Read the model definition and answer for the solid it produces. Units are mm, in the model's axes. A direction names the side the tool comes from. Coordinates: 2 decimals unless noted, no trailing zeros. Order: outer loops, then holes, each group sorted by start corner. A loop starts at its lowest first (then second) coordinate and runs counter-clockwise, first axis right, second up. Notation, with made-up numbers: (44, -15) - (99, -15) arc R21 ccw to (99, 1) - close; hole circle Ø5 at (-12, 15.5). An arc over 180 degrees is marked (long way). Use one line per item in the form item = value.
Autodesk Inventor part; units mm, degrees
ref_plane "YZ Plane" through (0, 0, 0) normal (1, 0, 0) x (0, 1, 0)
ref_plane "XZ Plane" through (0, 0, 0) normal (0, 1, 0) x (-1, 0, 0)
ref_plane "XY Plane" through (0, 0, 0) normal (0, 0, 1) x (1, 0, 0)
sketch "Sketch1" plane through (0, 0, 0) normal (0, 1, 0) x (-1, 0, 0)
  line L0 (0, 0) -> (-59, 0)
  line L1 (-59, 0) -> (-59, 5)
  line L2 (-59, 5) -> (0, 5)
  line L3 (0, 5) -> (0, 0)
  line L4 (0, 5) -> (-5, 5)
  line L5 (-5, 5) -> (-5, 47)
  line L6 (-5, 47) -> (0, 47)
  line L7 (0, 47) -> (0, 5)
  line L8 (-59, 5) -> (-54, 5)
  line L9 (-54, 5) -> (-54, 47)
  line L10 (-54, 47) -> (-59, 47)
  line L11 (-59, 47) -> (-59, 5)
  point P0 (-54, 5)
  dimension "d0" = 59
  dimension "d1" = 5
  dimension "d2" = 5
  dimension "d3" = 42
  dimension "d4" = 5
  dimension "d5" = 42
extrude "Extrusion1" add sketch "Sketch1" against normal blind 62
sketch "Sketch7" plane through (0, -62, 0) normal (0, -1, 0) x (1, 0, 0)
  line L0 (0, 47) -> (0, 0)
  line L1 (0, 47) -> (-5, 47)
  line L2 (-5, 47) -> (-5, -5)
  line L3 (-5, -5) -> (0, -5)
  line L4 (0, -5) -> (0, 47)
  line L5 (59, 47) -> (54, 47)
  line L6 (59, 47) -> (64, 47)
  line L7 (64, 47) -> (64, -5)
  line L8 (64, -5) -> (59, -5)
  line L9 (59, -5) -> (59, 47)
  line L10 (0, 0) -> (59, 0)
  line L11 (59, -5) -> (0, -5)
  line L12 (0, -5) -> (0, 0)
  line L13 (0, 0) -> (59, 0)
  line L14 (59, 0) -> (59, -5)
  dimension "d34" = 5
  dimension "d35" = 52
  dimension "d36" = 5
  dimension "d37" = 52
extrude "Extrusion7" add sketch "Sketch7" against normal blind 6
sketch "Sketch8" plane through (0, -62, 0) normal (0, -1, 0) x (1, 0, 0)
  line L0 (0, 0) -> (0, 47)
  line L1 (5, 47) -> (-5, 47)
  circle A0 centre (0, 37) radius 2.5
  line L2 (59, 47) -> (59, 0)
  line L3 (64, 47) -> (54, 47)
  circle A1 centre (59, 37) radius 2.5
  line L4 (59, 0) -> (0, 0)
  line L5 (-5, 47) -> (-5, -5)
  line L6 (64, -5) -> (64, 47)
  circle A2 centre (16.5, 0) radius 2.5
  circle A3 centre (42.5, 0) radius 2.5
  point P0 (29.5, 0)
  dimension "d40" = 10
  dimension "d41" = 5
  dimension "d42" = 10
  dimension "d43" = 5
  dimension "d44" = 34.5
  dimension "d47" = 5
  dimension "d48" = 5
  dimension "d56" = 13
  dimension "d57" = 13
extrude "Extrusion8" cut sketch "Sketch8" against normal blind 5
sketch "Sketch9" plane through (0, 0, 0) normal (-1, 0, 0) x (0, 0, 1)
  point P0 (0, 0)
sketch "Sketch10" plane through (0, 0, 0) normal (-1, 0, 0) x (0, 0, 1)
  line L0 (47, 0) -> (47, -56)
  line L1 (47, -62) -> (-5, -62)
  circle A0 centre (26, -12) radius 3
  point P0 (0, 0)
  dimension "d51" = 21
  dimension "d52" = 50
  dimension "d53" = 6
extrude "Extrusion9" cut sketch "Sketch10" against normal blind 5
equation "\"d4\" = d2"
equation "\"d5\" = d3"
equation "\"d43\" = d41"
equation "\"d47\" = d41"
equation "\"d48\" = d47"
properties part number "top cam mount v03"
(1) Section D-D, the plane x = 16.5 is taken. Write down the section's boundary in (y, z), then the cut area to 3 significant figures.
Answer list:
outline = (-62, -5) - (-56, -5) - (-56, 0) - (0, 0) - (0, 5) - (-62, 5) - (-62, 2.5) - (-57, 2.5) - (-57, -2.5) - (-62, -2.5) - close
area = 315 mm2
(2) Section A-A, the plane z = 37 is taken. Write down the section's boundary in (x, y).
Answer list:
outline = (-5, -62) - (-2.5, -62) - (-2.5, -57) - (2.5, -57) - (2.5, -62) - (5, -62) - (5, 0) - (0, 0) - (0, -56) - (-5, -56) - close; (54, -62) - (56.5, -62) - (56.5, -57) - (61.5, -57) - (61.5, -62) - (64, -62) - (64, -56) - (59, -56) - (59, 0) - (54, 0) - close
(3) Section B-B, the plane y = -25 is taken. Write down the section's boundary in (x, z), then the cut area to 3 significant figures.
Answer list:
outline = (0, 0) - (59, 0) - (59, 47) - (54, 47) - (54, 5) - (5, 5) - (5, 47) - (0, 47) - close
area = 715 mm2
(4) Which of the six approach directions +Z, -Z, +X, -X, +Y, -Y give full straight-line access (tool end or side, diameter ignored) to faces 4 (the flat face through (5, -31, 26)), 5 (the flat face through (2, -31, 47)), 6 (the cylindrical face through (2, -12, 23)), 7 (the flat face through (29, -28, 0)), 8 (the flat face through (59, -57, 37))?
Answer list:
face_4 = +Z, +Y, -Y
face_5 = +Z, +X, -X, +Y, -Y
face_6 = -X
face_7 = -Z, +X, -X, +Y
face_8 = -Y
(5) Section C-C, the plane z = 27 is taken. Write down the section's boundary in (x, y), then the cut area to 3 significant figures.
Answer list:
outline = (-5, -62) - (5, -62) - (5, -14.83) - (0, -14.83) - (0, -56) - (-5, -56) - close; (0, -9.17) - (5, -9.17) - (5, 0) - (0, 0) - close; (54, -62) - (64, -62) - (64, -56) - (59, -56) - (59, 0) - (54, 0) - close
area = 652 mm2
(6) The mould has two halves that part along X. Classify faces 1 (the flat face through (-5, -59, 21)), 2 (the flat face through (16, -57, 0)), 3 (the flat face through (30, -62, 4)): +X half, -X half, draft (parallel to the pull), parting line (faces both ways), or undercut.
Answer list:
face_1 = -X half
face_2 = undercut
face_3 = draft
(7) Straight lines are drawn through the part: L1, parallel to X at y = -59.25, z = 37; L2, parallel to X at y = -59.2, z = 0; L3, parallel to X at y = -17.5, z = 6. For each, find the intervals that lie inside material, in ascending order.
Answer list:
L1 = -5 to -2.5, 2.5 to 5, 54 to 56.5, 61.5 to 64
L2 = -5 to 14, 19 to 40, 45 to 64
L3 = 0 to 5, 54 to 59
(8) Given pin 1 Ø1.5 at (x, y) = (45.5, -31) entering from +Z; pin 2 Ø5 at (x, y) = (29.5, -10) entering from -Z; pin 3 Ø2.5 at (x, z) = (42, 1) entering from -Y, each flat-ended and moving along its own axis, determine where each tip first touches the part or whether it passes through.
Answer list:
pin_1 = 5
pin_2 = 0
pin_3 = -57
